For this review, use the dimensioned drawing (mm, ordinates from the lowest corner) and the shaded views. A direction names the side the tool comes from. Round coordinates to 2 decimals unless told otherwise and drop trailing zeros. Loops run counter-clockwise (first coordinate to the right, second up) from the corner with the lowest first, then second, coordinate; pieces in that order, holes last. Notation, with made-up numbers: (77, 80.5) -> (107, 80.5) arc R14 ccw to (107, 88.5) -> close; hole circle Ø10 at (32, 71.25). An arc over 180 degrees is marked (long way). Write each question's results on one line, items separated by ' | '.
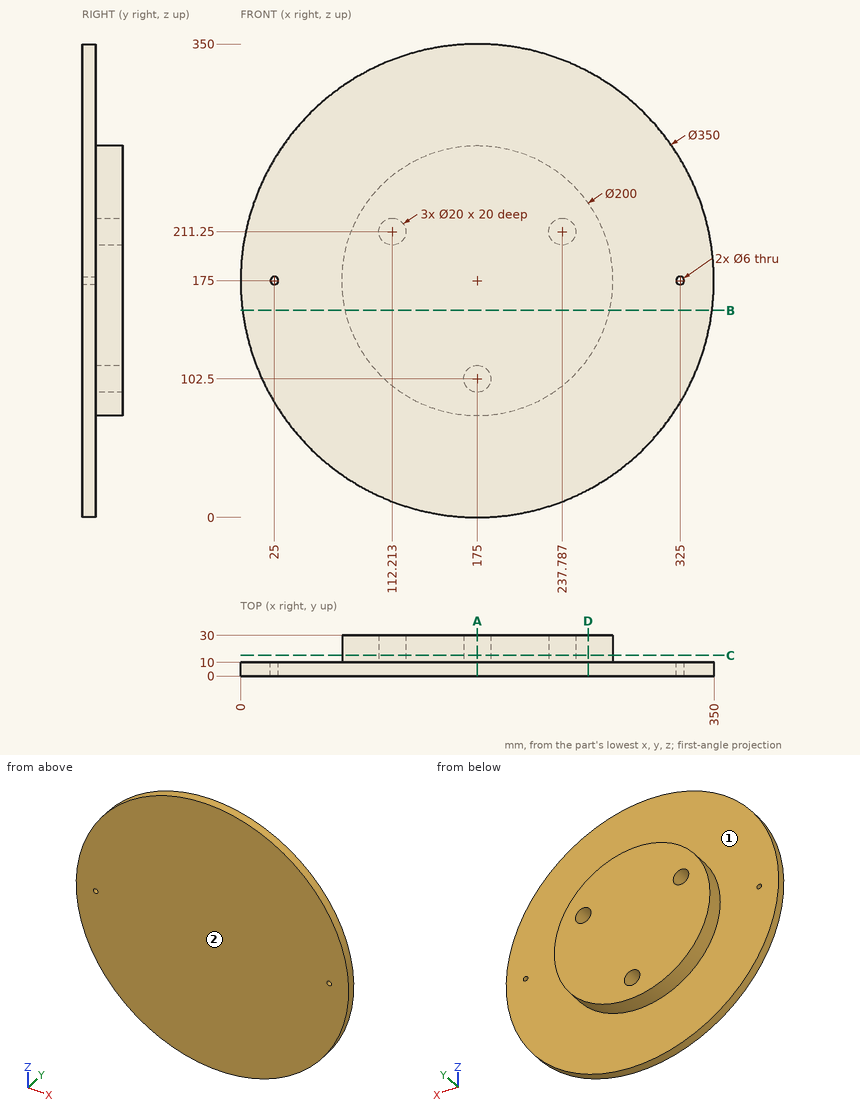
1. Consider section A-A (x = 175). State the section outline as (y, z) points.
Values found:
outline: (0, 0) -> (10, 0) -> (10, 75) -> (30, 75) -> (30, 92.5) -> (10, 92.5) -> (10, 112.5) -> (30, 112.5) -> (30, 275) -> (10, 275) -> (10, 350) -> (0, 350) -> close
2. Tool access review of the marked faces 1 and 2: name each direction out of +Z, -Z, +X, -X, +Y, -Y from which nothing blocks a thin tool from reaching the whole face with its end or side.
Values found:
face 1: +Y | face 2: +Z, -Z, +X, -X, -Y
3. Consider section D-D (x = 257). State the section outline as (y, z) points, plus the area to 3 significant figures.
Values found:
outline: (0, 20.4) -> (10, 20.4) -> (10, 117.76) -> (30, 117.76) -> (30, 232.24) -> (10, 232.24) -> (10, 329.6) -> (0, 329.6) -> close | area: 5,380 mm2
4. For pin 1 (6 mm diameter, centred on x = 233.5, z = 214, fed in from +Y); pin 2 (8 mm diameter, centred on y = 14.5, z = 136.5, fed in from +X); pin 3 (2 mm diameter, centred on y = 13.5, z = 189.5, fed in from -X), all flat-tipped, find the tip position at first contact; note any pin that passes through.
Values found:
pin 1: stops at y = 10 | pin 2: stops at x = 268.86 | pin 3: stops at x = 75.92
5. Consider section C-C (y = 15.25). State the section outline as (x, z) points.
Values found:
outline: circle Ø200 at (175, 175); hole circle Ø20 at (112.21, 211.25); hole circle Ø20 at (175, 102.5); hole circle Ø20 at (237.79, 211.25)
6. To check wall thickness, follow probe 1 along X at (y, z) = (2.5, 175); probe 2 along Y at (x, z) = (245.5, 98.5); probe 3 along X at (y, z) = (15.25, 211.25). State the ranges of each line that lie inside material, in increasing order.
Values found:
probe 1: x = 0 to 22, 28 to 322, 328 to 350 | probe 2: y = 0 to 10 | probe 3: x = 81.8 to 102.21, 122.21 to 227.79, 247.79 to 268.2
7. Consider section B-B (z = 153). State the section outline as (x, y) points, plus the area to 3 significant figures.
Values found:
outline: (1.39, 0) -> (348.61, 0) -> (348.61, 10) -> (272.55, 10) -> (272.55, 30) -> (77.45, 30) -> (77.45, 10) -> (1.39, 10) -> close | area: 7,370 mm2
